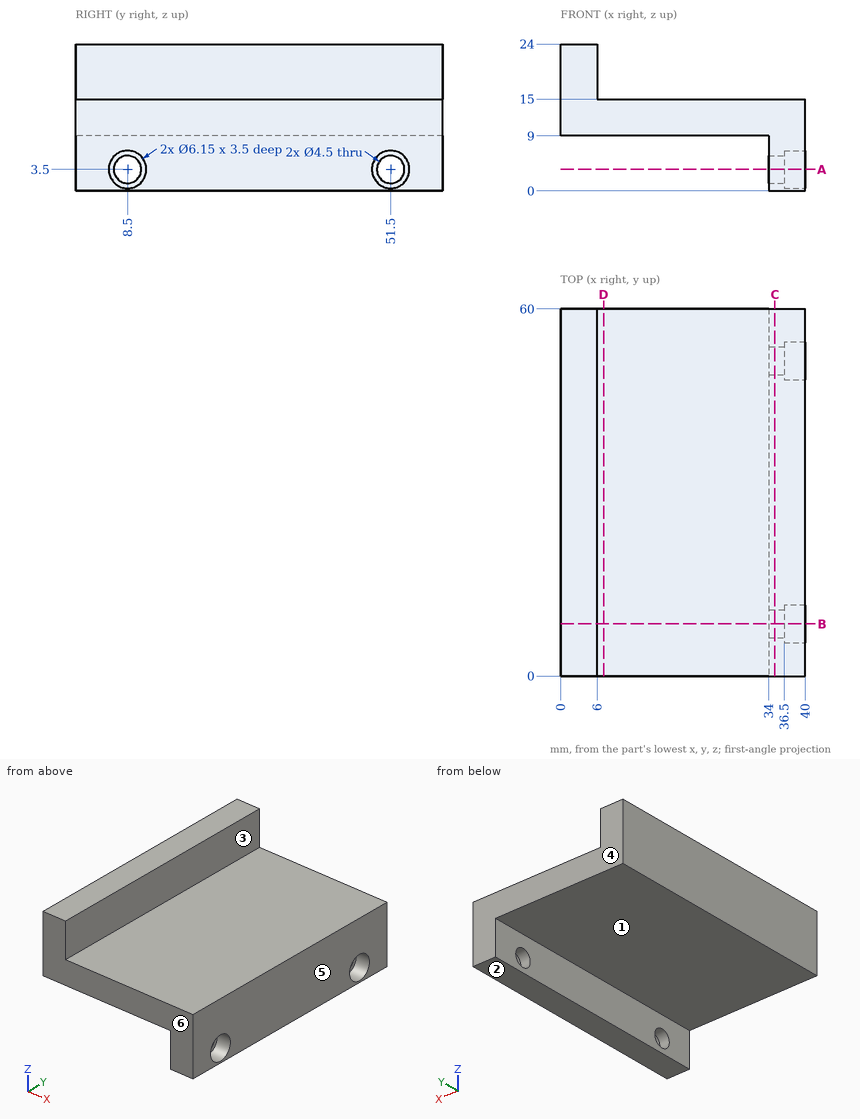
Design review of the part shown in the three views and the two pictorial views. Dimensions are in mm from the part's minimum x, y and z. A direction names the side the tool comes from. Round coordinates to 2 decimals unless told otherwise and drop trailing zeros. Loops run counter-clockwise (first coordinate to the right, second up) from the corner with the lowest first, then second, coordinate; pieces in that order, holes last. Notation, with made-up numbers: (58.5, 16.25) - (100.5, 16.25) arc R34 ccw to (100.5, 55.25) - close; hole circle Ø6 at (83, -37). An arc over 180 degrees is marked (long way). One line per item, written item: value. Start each with the question number.
Item 1: Clearance check with flat-ended pins moving along their axes: pin 1 Ø12 at (x, y) = (17, 15) entering from +Z; pin 2 Ø1 at (y, z) = (12, 17.5) entering from +X; pin 3 Ø5 at (y, z) = (8.5, 3.5) entering from -X; pin 4 Ø7 at (y, z) = (51.5, 3.5) entering from +X. State where each tip first meets the part, or that it passes through.
Item 2: Take a section at B-B (y = 8.5). Give the boundary of the cut face in (x, z) (3 decimals), plus the area to 3 significant figures.
Item 3: Take a section at C-C (x = 35). Give the boundary of the cut face in (y, z).
Item 4: Take a section at A-A (z = 3.5). Give the boundary of the cut face in (x, y) (3 decimals).
Item 5: For the marked faces 1, 2 and 3, list the 3-axis set-ups (+Z, -Z, +X, -X, +Y, -Y) from which the entire face can be reached by the end or side of a thin tool; tool diameter is ignored.
Item 6: For L1, parallel to Z at x = 39.25, y = 51.5 (3 decimals); L2, parallel to X at y = 38, z = 7.5; L3, parallel to Z at x = 37, y = 34.5, list the stretches that pass through material, from the lowest coordinate up.
Item 7: The part is to be moulded in two halves that separate along Y. For the marked faces 4, 5 and 6, say which applies: +Y half, -Y half, draft (parallel to the pull), parting line (faces both ways), or undercut.
Item 8: Take a section at D-D (x = 7). Give the boundary of the cut face in (y, z).
Answer below:
1. pin 1: stops at z = 15
1. pin 2: stops at x = 6
1. pin 3: stops at x = 34
1. pin 4: stops at x = 40
2. outline: (0, 9) - (34, 9) - (34, 5.75) - (36.5, 5.75) - (36.5, 6.575) - (40, 6.575) - (40, 15) - (6, 15) - (6, 24) - (0, 24) - close; (34, 0) - (40, 0) - (40, 0.425) - (36.5, 0.425) - (36.5, 1.25) - (34, 1.25) - close
2. area: 315 mm2
3. outline: (0, 0) - (60, 0) - (60, 15) - (0, 15) - close; hole circle Ø4.5 at (8.5, 3.5); hole circle Ø4.5 at (51.5, 3.5)
4. outline: (34, 0) - (40, 0) - (40, 5.425) - (36.5, 5.425) - (36.5, 6.25) - (34, 6.25) - close; (34, 10.75) - (36.5, 10.75) - (36.5, 11.575) - (40, 11.575) - (40, 48.425) - (36.5, 48.425) - (36.5, 49.25) - (34, 49.25) - close; (34, 53.75) - (36.5, 53.75) - (36.5, 54.575) - (40, 54.575) - (40, 60) - (34, 60) - close
5. face 1: -Z, -X, +Y, -Y
5. face 2: -Z, +X, -X, +Y, -Y
5. face 3: +Z, +X, +Y, -Y
6. L1: z = 0 to 0.425, 6.575 to 15
6. L2: x = 34 to 40
6. L3: z = 0 to 15
7. face 4: +Y half
7. face 5: draft
7. face 6: -Y half
8. outline: (0, 9) - (60, 9) - (60, 15) - (0, 15) - close
